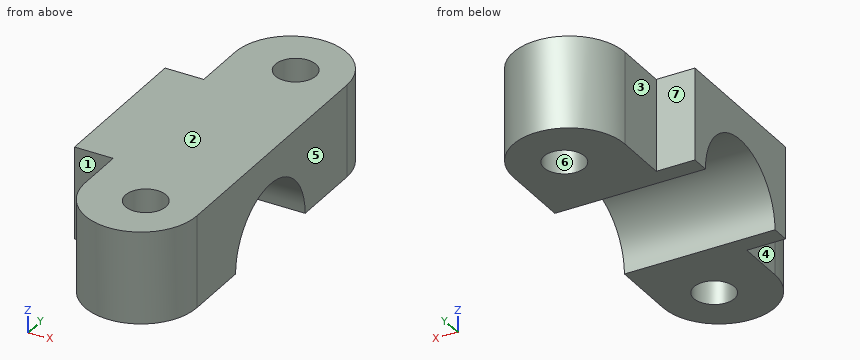
```python
from build123d import *

# Parameters (mm, degrees)
ESQUISSE1_R             = 1.1
EXTRUSION1_DEPTH        = 5
ESQUISSE2_R             = 3.25
ENL_V_MAT_EXTRU_1_DEPTH = 59.283442679


with BuildPart() as part:
    # Esquisse1 → Extrusion1 (new body)
    with BuildSketch(Plane.XY):
        with BuildLine():
            Line((-15.792310365, 40.455003044), (-15.792310365, 54.455003044))
            ThreePointArc((-15.792310365, 54.455003044), (-18.828177284, 57.490869963), (-21.864044203, 54.455003044))
            Line((-21.864044203, 54.455003044), (-21.864044203, 51.547447727))
            Line((-21.864044203, 51.547447727), (-23.962962816, 51.547447727))
            Line((-23.962962816, 51.547447727), (-23.962962816, 43.086270123))
            Line((-23.962962816, 43.086270123), (-21.864044203, 43.086270123))
            Line((-21.864044203, 43.086270123), (-21.864044203, 40.455003044))
            ThreePointArc((-21.864044203, 40.455003044), (-18.828177284, 37.419136124), (-15.792310365, 40.455003044))
        make_face()
        with Locations((-18.566221644, 40.455003043)):
            Circle(ESQUISSE1_R, mode=Mode.SUBTRACT)
        with Locations((-18.566221644, 54.455003043)):
            Circle(ESQUISSE1_R, mode=Mode.SUBTRACT)
    extrude(amount=EXTRUSION1_DEPTH)

    # Esquisse2 → Enlèv. mat.-Extru.1 (cut, through all)
    with BuildSketch(Plane.ZY.offset(23.962962816)):
        with Locations((0, 47.316858925)):
            Circle(ESQUISSE2_R)
    extrude(amount=-ENL_V_MAT_EXTRU_1_DEPTH, mode=Mode.SUBTRACT)


solid = part.part
```
Input: part model. Units: mm. Frame: model coordinates. Face numbers are marked on the shaded views. A direction names the side the tool comes from. Coordinates: 2 decimals unless noted, no trailing zeros. Loops run counter-clockwise (first coordinate to the right, second up) from the corner with the lowest first, then second, coordinate; pieces in that order, holes last. Notation, with made-up numbers: (45, 58.25) - (90, 58.25) arc R26 ccw to (90, 94.25) - close; hole circle Ø4 at (21, 80.25). An arc over 180 degrees is marked (long way). Answer in a Markdown table with one row per item.
(1) Mould query, pull axis X, two halves, no side actions, for the marked faces 4, 5, 6 and 7. Classes: pulls with the +X half, pulls with the -X half, needs draft (parallel to the pull), parting line crosses it, or undercut.
Model answer:
| item | result |
|---|---|
| face 4 | pulls with the -X half |
| face 5 | pulls with the +X half |
| face 6 | undercut |
| face 7 | needs draft |
(2) Cut plane A-A on z = 2.2. Output: boundary loops of the cut face in (x, y) (3 decimals), plus the area to 3 significant figures.
Model answer:
| item | result |
|---|---|
| outline | (-23.963, 43.086) - (-21.864, 43.086) - (-21.864, 40.455) arc R3.036 ccw to (-15.792, 40.455) - (-15.792, 44.925) - (-23.963, 44.925) - close; (-23.963, 49.709) - (-15.792, 49.709) - (-15.792, 54.455) arc R3.036 ccw to (-21.864, 54.455) - (-21.864, 51.547) - (-23.963, 51.547) - close; hole circle Ø2.2 at (-18.566, 40.455); hole circle Ø2.2 at (-18.566, 54.455) |
| area | 85.0 mm² |
(3) Pin query (flat end, axial travel): P1, Ø2.5, axis at x = -23.5, z = 2, coming from the -Y side; P2, Ø3, axis at y = 41.5, z = 3.5, coming from the -X side; P3, Ø1.3, axis at x = -18.57, y = 54.46, coming from the -Z side; P4, Ø0.6, axis at x = -22.5, z = 3, coming from the +Y side. Return the tip coordinate at first contact, or that it passes through.
Model answer:
| item | result |
|---|---|
| P1 | stops at y = 43.09 |
| P2 | stops at x = -21.86 |
| P3 | passes through |
| P4 | stops at y = 51.55 |
(4) Set-up query: the marked faces 1, 2 and 3. Return all of +Z, -Z, +X, -X, +Y, -Y with unobstructed straight access to the full face (end or side cutting, diameter ignored); none if empty.
Model answer:
| item | result |
|---|---|
| face 1 | +Z, -Z, -X, -Y |
| face 2 | +Z, +X, -X, +Y, -Y |
| face 3 | +Z, -Z, -X, +Y |
(5) Cut plane C-C on x = -19. Output: boundary loops of the cut face in (y, z), plus the area to 3 significant figures.
Model answer:
| item | result |
|---|---|
| outline | (37.42, 0) - (39.44, 0) - (39.44, 5) - (37.42, 5) - close; (41.47, 0) - (44.07, 0) arc R3.25 cw to (50.57, 0) - (53.44, 0) - (53.44, 5) - (41.47, 5) - close; (55.47, 0) - (57.49, 0) - (57.49, 5) - (55.47, 5) - close |
| area | 63.5 mm² |
(6) Cut plane B-B on y = 55. Output: boundary loops of the cut face in (x, z).
Model answer:
| item | result |
|---|---|
| outline | (-21.81, 0) - (-19.52, 0) - (-19.52, 5) - (-21.81, 5) - close; (-17.61, 0) - (-15.84, 0) - (-15.84, 5) - (-17.61, 5) - close |
(7) Material intervals for L1, parallel to Y at x = -19.25, z = 0.5; L2, parallel to Y at x = -18.75, z = 2.8; L3, parallel to X at y = 52.25, z = 4.85, sorted ascending. Write a range as from..to.
Model answer:
| item | result |
|---|---|
| L1 | y = 37.45..39.59, 41.32..44.11, 50.53..53.59, 55.32..57.46 |
| L2 | y = 37.42..39.37, 41.54..45.67, 48.97..53.37, 55.54..57.49 |
| L3 | x = -21.86..-15.79 |
(8) Cut plane D-D on z = 4.5. Output: boundary loops of the cut face in (x, y) (3 decimals).
Model answer:
| item | result |
|---|---|
| outline | (-23.963, 43.086) - (-21.864, 43.086) - (-21.864, 40.455) arc R3.036 ccw to (-15.792, 40.455) - (-15.792, 54.455) arc R3.036 ccw to (-21.864, 54.455) - (-21.864, 51.547) - (-23.963, 51.547) - close; hole circle Ø2.2 at (-18.566, 40.455); hole circle Ø2.2 at (-18.566, 54.455) |
